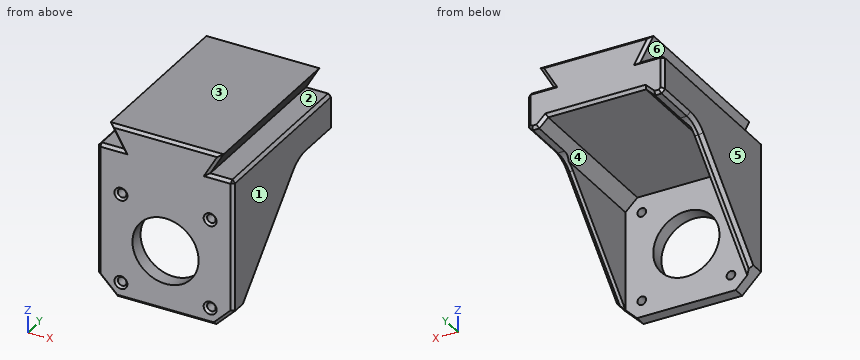
```python
from build123d import *

# Parameters (mm, degrees)
SKETCH1_R                       = 1.5
SKETCH1_R_2                     = 11.5
BRACKET_FACE_EXTRUDE_DEPTH      = 5
BRACKET_BODY_EXTRUDE_DEPTH      = 61
BRACKET_SIDE_TRIM_DEPTH         = 73.461334517
BRACKET_SIDE_TRIM_DEPTH_BACK    = 73.461334517
BRACKET_SIDE_EDGE_CHAMFER_SIZE  = 1.25
BRACKET_MOUNT_HOLE_CHAMFER_SIZE = 0.75
SLIDE_TAB_EXTRUDE_DEPTH         = 61
BRACKET_FACE_CHAMFER_SIZE       = 1


with BuildPart() as part:
    # Sketch1 → Bracket Face Extrude (new body)
    with BuildSketch(Plane(origin=(0, 0, 0), x_dir=(1, 0, 0), z_dir=(0, 1, 0))):
        Polygon((-21.15, 17.15), (-17.15, 21.15), (17.15, 21.15), (21.15, 17.15), (21.15, -17.15), (17, -21.15), (-17, -21.15), (-21.15, -17.15), align=None)
        with Locations(Location((-15.5, 15.5, 0), (0, 0, 270))):
            Circle(SKETCH1_R, mode=Mode.SUBTRACT)
        with Locations(Location((15.5, 15.5, 0), (0, 0, 270))):
            Circle(SKETCH1_R, mode=Mode.SUBTRACT)
        with Locations(Location((15.5, -15.5, 0), (0, 0, 270))):
            Circle(SKETCH1_R, mode=Mode.SUBTRACT)
        with Locations(Location((-15.5, -15.5, 0), (0, 0, 270))):
            Circle(SKETCH1_R, mode=Mode.SUBTRACT)
        with Locations(Location((0, 0, 0), (0, 0, 270))):
            Circle(SKETCH1_R_2, mode=Mode.SUBTRACT)
    extrude(amount=BRACKET_FACE_EXTRUDE_DEPTH)

    # Sketch5 → Bracket Body Extrude (add)
    with BuildSketch(Plane(origin=(0, 0, 0), x_dir=(1, 0, 0), z_dir=(0, 1, 0))):
        Polygon((-23.65, -18.212588103), (-23.65, -31.15), (23.65, -31.15), (23.65, -18.212588103), (23.65, 14.65), (21.15, 17.15), (21.15, -17.15), (17, -21.15), (-17, -21.15), (-21.15, -17.15), (-21.15, 17.15), (-23.65, 14.65), align=None)
    extrude(amount=BRACKET_BODY_EXTRUDE_DEPTH)

    # Sketch6 → Bracket Side Trim (cut, two sides: drawn at the far end of the back side and taken through both)
    with BuildSketch(Plane(origin=(0, 0, 0), x_dir=(0, 0, -1), z_dir=(1, 0, 0)).offset(-BRACKET_SIDE_TRIM_DEPTH_BACK)):
        with BuildLine():
            Line((17.15, 5), (-15.221067812, 37.371067812))
            ThreePointArc((-15.221067812, 37.371067812), (-17.388795325, 40.6153013), (-18.15, 44.442135624))
            Line((-18.15, 44.442135624), (-18.15, 61))
            Line((-18.15, 61), (17.15, 61))
            Line((17.15, 61), (17.15, 5))
        make_face()
    extrude(amount=BRACKET_SIDE_TRIM_DEPTH + BRACKET_SIDE_TRIM_DEPTH_BACK, mode=Mode.SUBTRACT)

    # Bracket Side Edge Chamfer
    bracket_side_edge_chamfer_edges = [part.edges().sort_by_distance(p)[0] for p in [
        (-23.65, 22.435533906, 0.285533906),
        (-23.65, 40.6153013, 17.388795325),
        (-23.65, 52.721067812, 18.15),
        (23.65, 52.721067812, 18.15),
        (23.65, 40.6153013, 17.388795325),
        (23.65, 22.435533906, 0.285533906),
    ]]
    chamfer(bracket_side_edge_chamfer_edges, length=BRACKET_SIDE_EDGE_CHAMFER_SIZE)

    # Bracket Mount Hole Chamfer
    bracket_mount_hole_chamfer_edges = [part.edges().sort_by_distance(p)[0] for p in [
        (-15.5, 0, -17),
        (15.5, 0, -17),
        (15.5, 0, 14),
        (-15.5, 0, 14),
    ]]
    chamfer(bracket_mount_hole_chamfer_edges, length=BRACKET_MOUNT_HOLE_CHAMFER_SIZE)

    # Sketch9 → Slide Tab Extrude (add)
    with BuildSketch(Plane(origin=(0, 0, 0), x_dir=(1, 0, 0), z_dir=(0, 1, 0))):
        Polygon((-15, -31.15), (-19.618802154, -39.15), (19.618802154, -39.15), (15, -31.15), align=None)
    extrude(amount=SLIDE_TAB_EXTRUDE_DEPTH)

    # Bracket Face Chamfer
    bracket_face_chamfer_edges = [part.edges().sort_by_distance(p)[0] for p in [
        (-23.65, 61, 25.275),
        (-21.25625, 61, 18.15),
        (23.025, 61, 18.775),
        (-23.025, 61, 18.775),
        (19.325, 0, 31.15),
        (19.325, 61, 31.15),
        (-17.309401077, 0, 35.15),
        (0, 0, 39.15),
        (17.309401077, 0, 35.15),
        (17.309401077, 61, 35.15),
        (-17.309401077, 61, 35.15),
        (0, 61, 39.15),
        (-23.65, 0, 8.25),
        (-19.325, 0, 31.15),
        (-23.65, 30.5, 31.15),
        (23.65, 0, 8.25),
        (23.65, 30.5, 31.15),
        (-19.325, 61, 31.15),
        (23.65, 61, 25.275),
        (0, 61, 21.15),
        (-18.55625, 61, 19.65),
        (18.55625, 61, 19.65),
        (21.25625, 61, 18.15),
        (-20.4, 0, -17.9),
        (0, 0, -21.15),
        (20.4, 0, -17.9),
    ]]
    chamfer(bracket_face_chamfer_edges, length=BRACKET_FACE_CHAMFER_SIZE)


solid = part.part
```
Geometry check sheet. Reference: the model listing, model coordinates, mm. Face numbers are marked on the shaded views. A direction names the side the tool comes from. Round coordinates to 2 decimals unless told otherwise and drop trailing zeros. Order: outer loops, then holes, each group sorted by start corner. A loop starts at its lowest first (then second) coordinate and runs counter-clockwise, first axis right, second up. Notation, with made-up numbers: (16, 35.5) - (34, 35.5) arc R14 ccw to (34, 44.5) - close; hole circle Ø6 at (-40, 36). An arc over 180 degrees is marked (long way). Use a Markdown table: item, result. Add a question column.
(1) Sectioned sample at C-C, the plane y = 35. Enter the section's corners in (x, z).
(2) Sectioned sample at D-D, the plane z = -9. Enter the section's corners in (x, y), and give its area (3 significant figures).
(3) Depth check by flat-ended pin: pin 1 (8.5 mm diameter, centred on x = -20, y = 16.5, fed in from +Z); pin 2 (1.1 mm diameter, centred on x = 21, y = 54.5, fed in from -Z). Enter the tip coordinate at first touch or a pass-through.
(4) Material ranges on line 1 along X through (y, z) = (3.7, 0); line 2 along X through (y, z) = (17, 17); line 3 along Z through (x, y) = (2, 40), recorded low to high. Write a range as [from, to].
(5) Sectioned sample at A-A, the plane x = 0. Enter the section's corners in (y, z), and give its area (3 significant figures).
(6) Sectioned sample at B-B, the plane z = 0. Enter the section's corners in (x, y).
(7) Tool access check on the marked faces 4, 5 and 6. Record the directions out of +Z, -Z, +X, -X, +Y, -Y that give a thin tool (end or side, any length) a straight path to the whole face; none if there is none.
(8) Release check for a two-part mould opening along Z. For the marked faces 1, 2 and 3 record: pulls with the +Z half, pulls with the -Z half, needs draft (parallel to the pull), parting line crosses it, or undercut.
Answers below:
| question | item | result |
|---|---|---|
| 1 | outline | (-23.65, 14.62) - (-22.4, 12.85) - (-21.15, 12.85) - (-21.15, 17.15) - (-17, 21.15) - (17, 21.15) - (21.15, 17.15) - (21.15, 12.85) - (22.4, 12.85) - (23.65, 14.62) - (23.65, 30.15) - (22.65, 31.15) - (15, 31.15) - (19.62, 39.15) - (-19.62, 39.15) - (-15, 31.15) - (-22.65, 31.15) - (-23.65, 30.15) - close |
| 2 | outline | (-23.65, 1) - (-22.65, 0) - (-7.16, 0) - (-7.16, 5) - (-21.15, 5) - (-21.15, 13.15) - (-22.4, 13.15) - (-23.65, 11.38) - close; (7.16, 0) - (22.65, 0) - (23.65, 1) - (23.65, 11.38) - (22.4, 13.15) - (21.15, 13.15) - (21.15, 5) - (7.16, 5) - close |
| 2 | area | 202 mm² |
| 3 | pin 1 | z = 39.15 |
| 3 | pin 2 | z = 18.15 |
| 4 | line 1 | [-23.65, -11.5], [11.5, 23.65] |
| 4 | line 2 | [-23.65, -21.15], [21.15, 23.65] |
| 4 | line 3 | [21.15, 39.15] |
| 5 | outline | (0, -20.15) - (1, -21.15) - (5, -21.15) - (5, -11.5) - (0, -11.5) - close; (0, 11.5) - (5, 11.5) - (5, 21.15) - (60, 21.15) - (61, 22.15) - (61, 38.15) - (60, 39.15) - (1, 39.15) - (0, 38.15) - close |
| 5 | area | 1,190 mm² |
| 6 | outline | (-23.65, 1) - (-22.65, 0) - (-11.5, 0) - (-11.5, 5) - (-21.15, 5) - (-21.15, 22.15) - (-22.4, 22.15) - (-23.65, 20.38) - close; (11.5, 0) - (22.65, 0) - (23.65, 1) - (23.65, 20.38) - (22.4, 22.15) - (21.15, 22.15) - (21.15, 5) - (11.5, 5) - close |
| 7 | face 4 | -Z, +Y |
| 7 | face 5 | +Z, -Z, -X, +Y, -Y |
| 7 | face 6 | -X, +Y, -Y |
| 8 | face 1 | needs draft |
| 8 | face 2 | undercut |
| 8 | face 3 | pulls with the +Z half |
